Here's how the part is built. I have some questions about the finished solid (model axes, mm). Face numbers are marked on the shaded views. A direction names the side the tool comes from. Round coordinates to 2 decimals unless told otherwise and drop trailing zeros. Write each loop counter-clockwise with the first axis right and the second up, starting at its lowest first coordinate (ties: lowest second). Pieces come first, ordered by that corner, then holes. Notation, with made-up numbers: (22.5, -26) - (33.5, -26) arc R12 ccw to (33.5, -18) - close; hole circle Ø1 at (-5, 23). An arc over 180 degrees is marked (long way). One line per item, written item: value. Start each with the question number.
Item 1: Imagine slicing it at A-A, the plane x = -6.35. Please give me the cut outline in (y, z) (3 decimals).
Item 2: Imagine slicing it at C-C, the plane z = 3.75. Please give me the cut outline in (x, y) (3 decimals), then the cut area to 3 significant figures.
Item 3: Thinking about a two-plate mould opening in X: for the marked faces 1 and 2, which applies, released by +X, released by -X, zero draft, split by the parting line, or undercut?
Item 4: If I drill on line 1 (Z direction, x = 3.25, y = -1) (3 decimals); line 2 (X direction, y = 1.75, z = -3.5); line 3 (X direction, y = 2, z = -3.5) (3 decimals), over which ranges is the centre line in solid material (lowest first)?
Item 5: For P1, Ø1, axis at x = 2.5, y = 4.5, coming from the -Z side (3 decimals); P2, Ø1, axis at y = 2, z = 0, coming from the +X side; P3, Ø1.5, axis at x = -4.5, z = -1.5, coming from the -Y side, each with a flat end and sliding along its axis, tell me the tip position at first contact or that it passes through.
Item 6: For the marked faces 3, 4, 5 and 6, which set-ups out of +Z, -Z, +X, -X, +Y, -Y let a thin tool reach every point of the face, with its end or its side?
Item 7: Imagine slicing it at D-D, the plane z = -5.75. Please give me the cut outline in (x, y) (3 decimals).
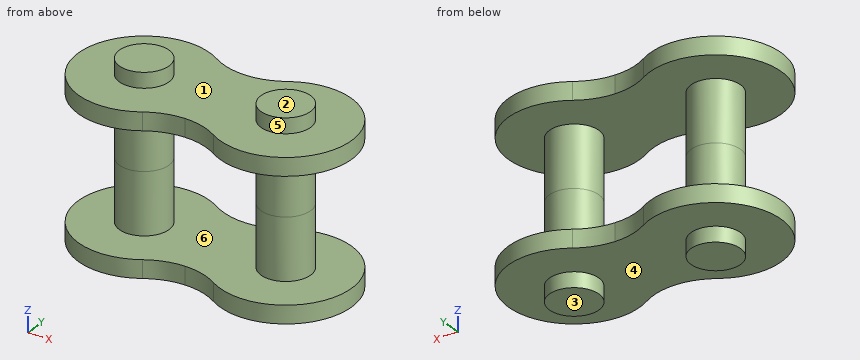
```python
from build123d import *

# Parameters (mm, degrees)
EXTRUDE_START   = -5.475
EXTRUDE_1_DEPTH = 1.6
SKETCH_1_3_R    = 2.225
EXTRUDE_2_DEPTH = 8.43


with BuildPart() as part:
    # Эскиз1 → Бобышка-Вытянуть1 (new body)
    with BuildSketch(Plane.XY.offset(EXTRUDE_START)):
        with BuildLine():
            Line((0, 4.045727726), (0, -4.045727726))
            ThreePointArc((0, -4.045727726), (-1.653799143, -4.282252786), (-3.175, -4.972863863))
            ThreePointArc((-3.175, -4.972863863), (-12.25, 0), (-3.175, 4.972863863))
            ThreePointArc((-3.175, 4.972863863), (-1.653799143, 4.282252786), (0, 4.045727726))
        make_face()
    extrude(amount=-EXTRUDE_1_DEPTH)

    # Эскиз1<3> → Бобышка-Вытянуть2 (add)
    with BuildSketch(Plane.XY):
        with Locations((-6.35, 0)):
            Circle(SKETCH_1_3_R)
    extrude(amount=-EXTRUDE_2_DEPTH)

    # Зеркальное отражение1: part across plane


with BuildPart() as part_1:
    add(part.part)
    add(part.part.mirror(Plane(origin=(0, 0, 0), x_dir=(0, 0, 1), z_dir=(1, 0, 0))))

    # Зеркальное отражение2: part across plane


with BuildPart() as part_2:
    add(part_1.part)
    add(part_1.part.mirror(Plane.XY))


solid = part_2.part
```
Values follow:
1. outline: (-5.9, -7.075) - (-2.225, -7.075) - (-2.225, -8.43) - (2.225, -8.43) - (2.225, -7.075) - (5.9, -7.075) - (5.9, -5.475) - (2.225, -5.475) - (2.225, 5.475) - (5.9, 5.475) - (5.9, 7.075) - (2.225, 7.075) - (2.225, 8.43) - (-2.225, 8.43) - (-2.225, 7.075) - (-5.9, 7.075) - (-5.9, 5.475) - (-2.225, 5.475) - (-2.225, -5.475) - (-5.9, -5.475) - close
2. outline: circle Ø4.45 at (-6.35, 0); circle Ø4.45 at (6.35, 0)
2. area: 31.1 mm^2
3. face 1: undercut
3. face 2: zero draft
4. line 1: z = -7.075 to -5.475, 5.475 to 7.075
4. line 2: x = -7.72 to -4.98, 4.98 to 7.72
4. line 3: x = -7.325 to -5.375, 5.375 to 7.325
5. P1: stops at z = -7.075
5. P2: stops at x = 7.99
5. P3: stops at y = -1.93
6. face 3: -Z, +X, -X, +Y, -Y
6. face 4: -Z
6. face 5: +Z
6. face 6: none
7. outline: (-3.175, -4.973) arc R5.9 cw to (3.175, -4.973) arc R5.9 ccw (long way) to (3.175, 4.973) arc R5.9 cw to (-3.175, 4.973) arc R5.9 ccw (long way) to start
